Part model, mm, in its own coordinate system. A direction names the side the tool comes from. Round coordinates to 2 decimals unless told otherwise and drop trailing zeros. Loops run counter-clockwise (first coordinate to the right, second up) from the corner with the lowest first, then second, coordinate; pieces in that order, holes last.
1) Mould opens along Y. For faces 3 (the cylindrical face through (93.782, 73.704, -16.367)), 4 (the conical face through (126.27, 12.24, -15.97)), 5 (the flat face through (190.226, -1, -32)) say: +Y half, -Y half, draft (parallel to the pull), parting line (faces both ways), or undercut.
2) 3-axis set-ups, long thin cutter, end or side, ignore diameter. For faces 1 (the flat face through (0, 56, 11)), 2 (the cylindrical face through (12.027, 50.125, 26.071)): which of +Z, -Z, +X, -X, +Y, -Y reach the whole face in a straight line?
3) Drop flat-ended pins along their axis: P1, Ø4, axis at x = 61, y = 30.5, coming from the +Z side; P2, Ø3, axis at x = 142.5, z = 12.5, coming from the +Y side; P3, Ø12, axis at x = 152.5, z = -47, coming from the +Y side; P4, Ø6, axis at y = -9, z = 27.5, coming from the +X side. Give the stop position or say it passes through.
4) Probe line 1 (Y direction, x = 8, z = 0); line 2 (Y direction, x = 133, z = 6); line 3 (Z direction, x = 155.5, y = 2). List the from-to ranges inside material, lowest first.
5) Band-saw the part on A-A, the plane z = -66. Write the cut outline in (x, y), then the cut area to 3 significant figures.
6) Band-saw the part on B-B, the plane z = 59. Write the cut outline in (x, y), then the cut area to 3 significant figures.
from build123d import *


with BuildPart() as part:
    # Model → Revolve1 (revolve)
    with BuildSketch(Plane.XY, mode=Mode.PRIVATE) as revolve1_sk:
        with BuildLine():
            Line((0, 56.499761536), (23.721747443, 56.499761536))
            ThreePointArc((23.721747443, 56.499761536), (61.910828562, 51.472073195), (97.497386789, 36.731637642))
            Line((97.497386789, 36.731637642), (131.736780289, 16.963514588))
            ThreePointArc((131.736780289, 16.963514588), (136.846780231, 14.84688352), (142.330485577, 14.124940199))
            ThreePointArc((142.330485577, 14.124940199), (143.215010337, 14.197934269), (144.075603175, 14.414941534))
            add(Edge.make_bspline(
                [(144.075603175, 14.414941534), (185.934060843, 28.722002721), (190.226374917, 30.032918805)],
                knots=[0, 0, 0, 1, 1, 1], degree=2))
            Line((190.226374917, 30.032918805), (190.226374917, 75.499761536))
            Line((190.226374917, 75.499761536), (0, 75.499761536))
            Line((0, 75.499761536), (0, 56.499761536))
        make_face()
    revolve(revolve1_sk.sketch.rotate(Axis((0, 0, 0), (1, 0, 0)), 90), axis=Axis((0, 0, 0), (1, 0, 0)))


solid = part.part
Reported:
1. face 3: parting line
1. face 4: undercut
1. face 5: draft
2. face 1: +Z, -Z, -X, +Y, -Y
2. face 2: -X
3. P1: stops at z = 69.91
3. P2: stops at y = 74.69
3. P3: stops at y = 63.4
3. P4: stops at x = 190.23
4. line 1: y = -75.5 to -56.5, 56.5 to 75.5
4. line 2: y = -75.26 to -15.14, 15.14 to 75.26
4. line 3: z = -75.47 to -18.21, 18.21 to 75.47
5. outline: (0, -36.66) - (190.23, -36.66) - (190.23, 36.66) - (0, 36.66) - close
5. area: 13,900 mm2
6. outline: (0, -47.11) - (190.23, -47.11) - (190.23, 47.11) - (0, 47.11) - close
6. area: 17,900 mm2
